from build123d import *

# Parameters (mm, degrees)
BOSS_EXTRUDE1_DEPTH = 2405.888
SKETCH3_W           = 108.204
SKETCH3_H           = 91.948
CUT_EXTRUDE1_DEPTH  = 50.8
SKETCH4_R           = 50.8
CUT_EXTRUDE2_DEPTH  = 25.4


with BuildPart() as part:
    # Sketch2 → Boss-Extrude1 (new body)
    with BuildSketch(Plane(origin=(0, 0, 0), x_dir=(1, 0, 0), z_dir=(0, 1, 0))):
        Polygon((-457.073, 291.592), (-428.625, 291.592), (-428.625, 0), (428.625, 0), (428.625, 291.592), (727.075, 291.592), (727.075, 240.792), (454.025, 240.792), (454.025, -25.4), (-457.073, -25.4), align=None)
    extrude(amount=BOSS_EXTRUDE1_DEPTH)

    # Sketch3 → Cut-Extrude1 (cut)
    with BuildSketch(Plane.XY.offset(-240.792)):
        with Locations((672.973, 2359.914)):
            Rectangle(SKETCH3_W, SKETCH3_H)
    extrude(amount=-CUT_EXTRUDE1_DEPTH, mode=Mode.SUBTRACT)

    # Sketch4 → Cut-Extrude2 (cut)
    with BuildSketch(Plane.XY.offset(25.4)):
        with Locations((-365.125, 2235.708)):
            Circle(SKETCH4_R)
    extrude(amount=-CUT_EXTRUDE2_DEPTH, mode=Mode.SUBTRACT)


solid = part.part
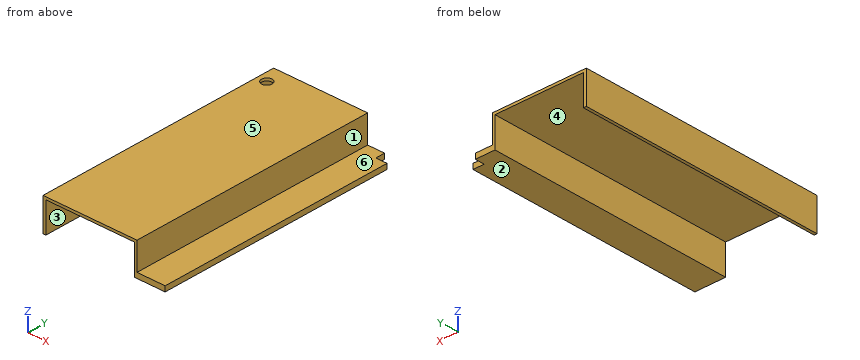
Read the model definition and answer for the solid it produces. Units are mm, in the model's axes. Face numbers are marked on the shaded views. A direction names the side the tool comes from. Round coordinates to 2 decimals unless told otherwise and drop trailing zeros. Loops run counter-clockwise (first coordinate to the right, second up) from the corner with the lowest first, then second, coordinate; pieces in that order, holes last.
Q1. Section D-D on x = 546 is taken. Write down the section's boundary in (y, z).
Q2. Each of these flat-tipped pins is pushed along its axis until it touches: pin 1 (6 mm diameter, centred on x = 175, y = 1941.5, fed in from -Z); pin 2 (6 mm diameter, centred on y = 526, z = -48.5, fed in from +X) (3 decimals). Where does it stop, or does it pass through?
Q3. Consider probe 1 along X at (y, z) = (104.5, -180) (3 decimals); probe 2 along X at (y, z) = (1866.5, -266.5) (3 decimals); probe 3 along Z at (x, y) = (-346, 2000). Determine where each line is inside the solid, lowest interval first.
Q4. Section A-A on z = -156 is taken. Write down the section's boundary in (x, y) (3 decimals), and give its area (3 significant figures).
Q5. Determine the mould class of the marked faces 1, 2 and 3 for opening direction X: released by +X, released by -X, zero draft, split by the parting line, or undercut.
Q6. Section C-C on x = -135.5 is taken. Write down the section's boundary in (y, z), and give its area (3 significant figures).
Q7. Section B-B on y = 765.5 is taken. Write down the section's boundary in (x, z) (3 decimals), and give its area (3 significant figures).
Q8. Which of the six approach directions +Z, -Z, +X, -X, +Y, -Y give full straight-line access (tool end or side, diameter ignored) to the marked faces 4, 5 and 6?
Output:
1. outline: (0, -291.59) - (2405.89, -291.59) - (2405.89, -240.79) - (0, -240.79) - close
2. pin 1: stops at z = 0
2. pin 2: stops at x = 454.025
3. probe 1: x = -457.073 to -428.625, 428.625 to 454.025
3. probe 2: x = -457.073 to -428.625, 428.625 to 727.075
3. probe 3: z = 0 to 25.4
4. outline: (-457.073, 0) - (-428.625, 0) - (-428.625, 2405.888) - (-457.073, 2405.888) - close; (428.625, 0) - (454.025, 0) - (454.025, 2405.888) - (428.625, 2405.888) - close
4. area: 130,000 mm2
5. face 1: released by +X
5. face 2: zero draft
5. face 3: undercut
6. outline: (0, 0) - (2405.89, 0) - (2405.89, 25.4) - (0, 25.4) - close
6. area: 61,100 mm2
7. outline: (-457.073, -291.592) - (-428.625, -291.592) - (-428.625, 0) - (428.625, 0) - (428.625, -291.592) - (727.075, -291.592) - (727.075, -240.792) - (454.025, -240.792) - (454.025, 25.4) - (-457.073, 25.4) - close
7. area: 52,700 mm2
8. face 4: -Z, +Y, -Y
8. face 5: +Z, +X, -X, +Y, -Y
8. face 6: +Z, +X, +Y, -Y
